Verification items for this drawing (mm, ordinates from the low corner). Coordinates: 2 decimals unless noted, no trailing zeros. Order: outer loops, then holes, each group sorted by start corner. A loop starts at its lowest first (then second) coordinate and runs counter-clockwise, first axis right, second up. Notation, with made-up numbers: M -10.75,55.25 L 11.25,55.25 A17 cw 11.25,88.25 Z; hole C 76.25,-2.5 d5. An arc over 180 degrees is marked long. Answer as a JSON object with one key per item and string values. Group by question number.
(1) Mould release check, pull along X, two halves, no side actions. Record for the marked faces 1 and 2: released by +X, released by -X, zero draft, split by the parting line, or undercut.
(2) Cross-section at B-B (x = 22.25). Enter the section's corners in (y, z), plus the area to 3 significant figures.
(3) Material ranges on line 1 (Y direction, x = 2.5, z = 0.7); line 2 (Y direction, x = 22, z = 1.5); line 3 (Z direction, x = 10.5, y = 5.5), recorded low to high.
(4) Gauge pin test, flat ends, axial feed: pin 1 Ø2 at (x, y) = (2.5, 35) entering from -Z; pin 2 Ø5 at (x, y) = (17.5, 22.5) entering from +Z. Record the tip position at first contact, or that the pin passes through.
(5) Cross-section at D-D (y = 24.75). Enter the section's corners in (x, z), plus the area to 3 significant figures.
(6) Cross-section at C-C (z = 0.65). Count the separate pieces of the cut face and the enclosed holes in it, plus the area to 3 significant figures.
(7) Cross-section at A-A (y = 5). Enter the section's corners in (x, z), plus the area to 3 significant figures.
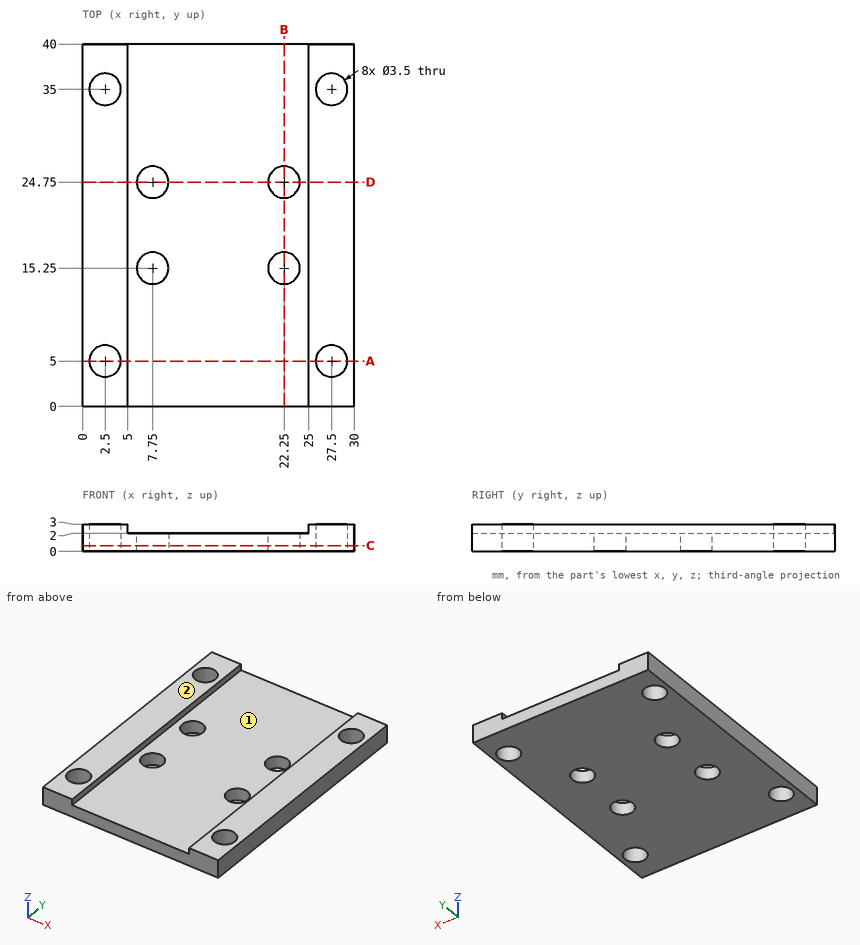
Taken from the geometry:
{
 "1": {"face 1": "undercut", "face 2": "zero draft"},
 "2": {"outline": "M 0,0 L 13.5,0 L 13.5,2 L 0,2 Z; M 17,0 L 23,0 L 23,2 L 17,2 Z; M 26.5,0 L 40,0 L 40,2 L 26.5,2 Z", "area": "66.0 mm²"},
 "3": {"line 1": "y = 0 to 3.25, 6.75 to 33.25, 36.75 to 40", "line 2": "y = 0 to 13.52, 16.98 to 23.02, 26.48 to 40", "line 3": "z = 0 to 2"},
 "4": {"pin 1": "passes through", "pin 2": "stops at z = 2"},
 "5": {"outline": "M 0,0 L 6,0 L 6,2 L 5,2 L 5,3 L 0,3 Z; M 9.5,0 L 20.5,0 L 20.5,2 L 9.5,2 Z; M 24,0 L 30,0 L 30,3 L 25,3 L 25,2 L 24,2 Z", "area": "56.0 mm²"},
 "6": {"separate pieces": "1", "enclosed holes": "8", "area": "1,120 mm²"},
 "7": {"outline": "M 0,0 L 0.75,0 L 0.75,3 L 0,3 Z; M 4.25,0 L 25.75,0 L 25.75,3 L 25,3 L 25,2 L 5,2 L 5,3 L 4.25,3 Z; M 29.25,0 L 30,0 L 30,3 L 29.25,3 Z", "area": "49.0 mm²"}
}
